from build123d import *

# Parameters (mm, degrees)
SZKIC1_W                    = 9.5
SZKIC1_H                    = 36
DODANIE_WYCI_GNI_CIE1_DEPTH = 9.9
SZKIC2_W                    = 7
SZKIC2_H                    = 23.5
WYTNIJ_WYCI_GNI_CIE1_DEPTH  = 9.9
SZKIC3_R                    = 2.5
DODANIE_WYCI_GNI_CIE2_DEPTH = 7.5
WYTNIJ_WYCI_GNI_CIE2_DEPTH  = 137.5
WYTNIJ_WYCI_GNI_CIE3_DEPTH  = 137.5
ZAOKR_GLENIE1_R             = 10
ZAOKR_GLENIE2_R             = 2
SZKIC6_R                    = 3.75
WYTNIJ_WYCI_GNI_CIE4_DEPTH  = 10


with BuildPart() as part:
    # Szkic1 → Dodanie-wyciągnięcie1 (new body)
    with BuildSketch(Plane.XY):
        with Locations((-4.75, 18)):
            Rectangle(SZKIC1_W, SZKIC1_H)
    extrude(amount=DODANIE_WYCI_GNI_CIE1_DEPTH)

    # Szkic2 → Wytnij-wyciągnięcie1 (cut)
    with BuildSketch(Plane.XY.offset(9.9)):
        with Locations((-3.5, 17.25)):
            Rectangle(SZKIC2_W, SZKIC2_H)
    extrude(amount=-WYTNIJ_WYCI_GNI_CIE1_DEPTH, mode=Mode.SUBTRACT)

    # Szkic3 → Dodanie-wyciągnięcie2 (add)
    with BuildSketch(Plane.ZY.offset(9.5)):
        with BuildLine():
            Line((7.4, 36), (9.9, 36))
            Line((9.9, 36), (12.4, 32.923076923))
            Line((12.4, 32.923076923), (29.4, 12))
            Line((29.4, 12), (31.9, -4))
            ThreePointArc((31.9, -4), (26.9, -9), (21.9, -4))
            Line((21.9, -4), (21.9, 0))
            Line((21.9, 0), (12.4, 0))
            Line((12.4, 0), (7.4, 0))
            Line((7.4, 0), (7.4, 36))
        make_face()
        with Locations((26.9, -4)):
            Circle(SZKIC3_R, mode=Mode.SUBTRACT)
    extrude(amount=DODANIE_WYCI_GNI_CIE2_DEPTH)

    # Szkic4 → Wytnij-wyciągnięcie2 (cut)
    with BuildSketch(Plane(origin=(0, 36, 0), x_dir=(1, 0, 0), z_dir=(0, 1, 0))):
        Polygon((-12, -7.4), (-22.251097051, -17.651097051), (-26.525986736, -7.4), align=None)
        Polygon((-10.964466094, -9.9), (-14.5, -13.435533906), (-14.5, -34.97095788), (-2.856589665, -34.97095788), (-4.384348652, -9.9), align=None)
    extrude(amount=-WYTNIJ_WYCI_GNI_CIE2_DEPTH, mode=Mode.SUBTRACT)

    # Szkic5 → Wytnij-wyciągnięcie3 (cut)
    with BuildSketch(Plane.ZY.offset(17)):
        with BuildLine():
            Line((14.930271414, 20.050399523), (21.630271414, 12.888330558))
            ThreePointArc((21.630271414, 12.888330558), (21.830126715, 12.572412171), (21.9, 12.205173429))
            Line((21.9, 12.205173429), (21.9, 7.1))
            ThreePointArc((21.9, 7.1), (21.607106781, 6.392893219), (20.9, 6.1))
            Line((20.9, 6.1), (14.2, 6.1))
            ThreePointArc((14.2, 6.1), (13.492893219, 6.392893219), (13.2, 7.1))
            Line((13.2, 7.1), (13.2, 19.367242395))
            ThreePointArc((13.2, 19.367242395), (13.832761259, 20.29736911), (14.930271414, 20.050399523))
        make_face()
    extrude(amount=-WYTNIJ_WYCI_GNI_CIE3_DEPTH, mode=Mode.SUBTRACT)

    # Zaokrąglenie1
    zaokr_glenie1_edges = [part.edges().sort_by_distance(p)[0] for p in [
        (-15.75, 12, 29.4),
    ]]
    fillet(zaokr_glenie1_edges, radius=ZAOKR_GLENIE1_R)

    # Zaokrąglenie2
    zaokr_glenie2_edges = [part.edges().sort_by_distance(p)[0] for p in [
        (-15.75, 0, 21.9),
    ]]
    fillet(zaokr_glenie2_edges, radius=ZAOKR_GLENIE2_R)

    # Szkic6 → Wytnij-wyciągnięcie4 (cut)
    with BuildSketch(Plane.ZY.offset(17)):
        with Locations((26.9, -4)):
            Circle(SZKIC6_R)
    extrude(amount=-WYTNIJ_WYCI_GNI_CIE4_DEPTH, mode=Mode.SUBTRACT)


solid = part.part
Check sheet for the modelled part. Datum: model origin and axes. Units: mm. A direction names the side the tool comes from. Round coordinates to 2 decimals unless told otherwise and drop trailing zeros. Order: outer loops, then holes, each group sorted by start corner. A loop starts at its lowest first (then second) coordinate and runs counter-clockwise, first axis right, second up.
(1) Cross-section at C-C, the plane y = 8. Enter the section's corners in (x, z) (3 decimals).
(2) Go/stop test with flat-tipped pins: P1, Ø4, axis at y = 7.5, z = 7.5, coming from the -X side; P2, Ø0.8, axis at x = -11.5, y = 11, coming from the -Z side; P3, Ø3.5, axis at y = 19.5, z = 5.5, coming from the -X side. Record where each tip stops, or that it passes through.
(3) Access from +Z, -Z, +X, -X, +Y, -Y to the whole of each face (thin tool, end or side, straight path). Record for faces 5 (the flat face through (-4, 29, 5)), 6 (the flat face through (-15.768, 16.519, 18.233)), 7 (the flat face through (-7, 0, 7)).
(4) Cross-section at D-D, the plane z = 26.9. Enter the section's corners in (x, y).
(5) Cross-section at A-A, the plane x = -6.25. Enter the section's corners in (y, z), and give its area (3 significant figures).
(6) Scan lines: probe 1 along Z at (x, y) = (-1.5, 1); probe 2 along Y at (x, z) = (-14.75, 25.5); probe 3 along Y at (x, z) = (-9, 9). Record each from-to range of solid material in increasing order.
(7) Draft check along Z on faces 1 (the cylindrical face through (-15.768, 6.401, 21.615)), 2 (the flat face through (-11, 18, 7.4)), 3 (the cylindrical face through (-16, -9, 27)), 4 (the flat face through (-8, 18, 9.9)). Enter one of: pulls with the +Z half, pulls with the -Z half, needs draft (parallel to the pull), parting line crosses it, or undercut.
(8) Cross-section at B-B, the plane z = 6. Enter the section's corners in (x, y).
Check sheet entries:
1. outline: (-17, 12.4) - (-12, 7.4) - (-9.5, 7.4) - (-9.5, 0) - (-7, 0) - (-7, 9.9) - (-10.964, 9.9) - (-14.264, 13.2) - (-17, 13.2) - close; (-17, 21.9) - (-14.5, 21.9) - (-14.5, 30.025) - (-17, 30.025) - close
2. P1: stops at x = -14.1
2. P2: stops at z = 7.4
2. P3: stops at x = -9.5
3. face 5: +Z, -Z, +X
3. face 6: +X, -X
3. face 7: -Z, +X, -X, -Y
4. outline: (-17, -9) - (-14.5, -9) - (-14.5, -7.75) - (-17, -7.75) - close; (-17, -0.25) - (-14.5, -0.25) - (-14.5, 15.08) - (-17, 15.08) - close
5. outline: (0, 0) - (5.5, 0) - (5.5, 9.9) - (0, 9.9) - close; (29, 0) - (36, 0) - (36, 9.9) - (29, 9.9) - close
5. area: 124 mm2
6. probe 1: z = 0 to 9.9
6. probe 2: y = -8.8 to -7.48, -0.52 to 16.8
6. probe 3: y = 0 to 36
7. face 1: undercut
7. face 2: pulls with the -Z half
7. face 3: parting line crosses it
7. face 4: pulls with the +Z half
8. outline: (-9.5, 0) - (0, 0) - (0, 5.5) - (-7, 5.5) - (-7, 29) - (0, 29) - (0, 36) - (-9.5, 36) - close
